Input: part model. Units: mm. Frame: model coordinates. A direction names the side the tool comes from. Give positions to 0.01 mm unless a question says otherwise; leave off trailing zeros. Loops run counter-clockwise (first coordinate to the right, second up) from the corner with the lowest first, then second, coordinate; pieces in that order, holes last. Notation, with made-up numbers: (19.5, 64) - (53.5, 64) arc R12 ccw to (53.5, 77) - close; hole circle Ø11 at (48, 52). An arc over 180 degrees is marked (long way). Answer as a JSON object with one key per item and string values. Group by question number.
(1) Access query for faces 4 (the cylindrical face through (-42.19, 15.07, -8.69)), 5 (the flat face through (-42, 15, 12)), 6 (the flat face through (-1, 2.5, 16)), 7 (the flat face through (27, 13.05, -27)). Directions: +Z, -Z, +X, -X, +Y, -Y. A direction counts if a zero-diameter tool reaches every point of the face in a straight line with its end or side. Return the directions, or none.
(2) Mould query, pull axis X, two halves, no side actions, for faces 1 (the flat face through (0, 6.5, 39)), 2 (the cylindrical face through (0.352, 14.93, -54.496)), 3 (the cylindrical face through (38.845, 7.918, -17.093)). Classes: +X half, -X half, draft (parallel to the pull), parting line (faces both ways), or undercut.
(3) Material intervals for L1, parallel to Z at x = 0, y = 1; L2, parallel to Z at x = -2, y = 18.25; L3, parallel to X at y = 9, z = 13, sorted ascending.
(4) Section query A-A (x = 0). Return loops of the section in (y, z).
(5) Section query B-B (z = -3.5). Return loops of the section in (x, y).
(6) Pin query (flat end, axial travel): P1, Ø2, axis at y = 11, z = -22, coming from the -X side; P2, Ø3, axis at x = 31, y = 15, coming from the +Z side; P3, Ø7.5, axis at x = 46, z = -6, coming from the -Y side. Return the tip coordinate at first contact, or that it passes through.
(7) Section query C-C (y = 5). Count the separate pieces of the cut face and the enclosed holes in it, plus the area to 3 significant figures.
```python
from build123d import *

# Parameters (mm, degrees)
BOSS_EXTRUDE1_DEPTH = 20
SKETCH5_W           = 4
SKETCH5_H           = 10
SKETCH16_W          = 2
SKETCH16_H          = 4.5
CUT_EXTRUDE9_DEPTH  = 10
SKETCH19_W          = 4
SKETCH19_H          = 10
CUT_EXTRUDE4_DEPTH  = 17.5
CUT_EXTRUDE5_DEPTH  = 2.5
SKETCH15_W          = 11.5
SKETCH15_H          = 4.5
CUT_EXTRUDE8_DEPTH  = 2.5
SKETCH17_W          = 14
SKETCH17_H          = 3
CUT_EXTRUDE10_DEPTH = 2.5
SKETCH21_W          = 4.5
SKETCH21_H          = 2
CUT_EXTRUDE11_DEPTH = 10
SKETCH22_R          = 2
CUT_EXTRUDE12_DEPTH = 2.5
FILLET1_R           = 10
FILLET2_R           = 4
SKETCH24_W          = 4.1
SKETCH24_H          = 4
CUT_EXTRUDE14_DEPTH = 77.5
SKETCH28_W          = 4.1
SKETCH28_H          = 4
CUT_EXTRUDE15_DEPTH = 77.5
SKETCH23_R          = 22.75
CUT_EXTRUDE13_DEPTH = 2.5


with BuildPart() as part:
    # Sketch1 → Boss-Extrude1 (new body)
    with BuildSketch(Plane(origin=(0, 0, 0), x_dir=(1, 0, 0), z_dir=(0, 1, 0))):
        Polygon((16.568542495, 40), (-16.568542495, 40), (-40, 16.568542495), (-40, -16.568542495), (-16.568542495, -40), (16.568542495, -40), (40, -16.568542495), (40, 16.568542495), align=None)
    extrude(amount=BOSS_EXTRUDE1_DEPTH)

    # Sweep9: sweep along a path in Sketch7
    with BuildLine(Plane(origin=(0, 15, 0), x_dir=(1, 0, 0), z_dir=(0, 1, 0))) as sweep9_path:
        ThreePointArc((40, -10.5), (50.5, 0), (40, 10.5))
    # Sketch5 → Sweep9 (sweep)
    with BuildSketch(Plane(origin=(40, 0, 0), x_dir=(0, 0, -1), z_dir=(1, 0, 0))):
        with Locations((-12.5, 15)):
            Rectangle(SKETCH5_W, SKETCH5_H)
        with Locations((12.5, 15)):
            Rectangle(SKETCH5_W, SKETCH5_H)
    sweep9 = sweep(path=sweep9_path.line)

    # Sketch16 → Cut-Extrude9 (cut)
    with BuildSketch(Plane(origin=(0, 20, 0), x_dir=(1, 0, 0), z_dir=(0, 1, 0))):
        with Locations((41, -12.25)):
            Rectangle(SKETCH16_W, SKETCH16_H)
    cut_extrude9 = extrude(amount=-CUT_EXTRUDE9_DEPTH, mode=Mode.SUBTRACT)

    # Mirror1: Sweep9, Cut-Extrude9 across plane
    add(sweep9.mirror(Plane(origin=(0, 0, 0), x_dir=(0, 0, 1), z_dir=(1, 0, 0))))
    add(cut_extrude9.mirror(Plane(origin=(0, 0, 0), x_dir=(0, 0, 1), z_dir=(1, 0, 0))), mode=Mode.SUBTRACT)

    # Sweep10: sweep along a path in Sketch20
    with BuildLine(Plane(origin=(0, 15, 0), x_dir=(1, 0, 0), z_dir=(0, 1, 0))) as sweep10_path:
        ThreePointArc((10.5, 40), (0, 50.5), (-10.5, 40))
    # Sketch19 → Sweep10 (sweep)
    with BuildSketch(Plane(origin=(0, 0, -40), x_dir=(-1, 0, 0), z_dir=(0, 0, -1))):
        with Locations((-12.5, 15)):
            Rectangle(SKETCH19_W, SKETCH19_H)
        with Locations((12.5, 15)):
            Rectangle(SKETCH19_W, SKETCH19_H)
    sweep(path=sweep10_path.line)

    # Sketch6 → Cut-Extrude4 (cut)
    with BuildSketch(Plane(origin=(0, 20, 0), x_dir=(1, 0, 0), z_dir=(0, 1, 0))):
        Polygon((-15.533008589, -37.5), (15.533008589, -37.5), (37.5, -15.533008589), (37.5, 15.533008589), (15.533008589, 37.5), (-15.533008589, 37.5), (-37.5, 15.533008589), (-37.5, -15.533008589), align=None)
    extrude(amount=-CUT_EXTRUDE4_DEPTH, mode=Mode.SUBTRACT)

    # Sketch3 → Cut-Extrude5 (cut)
    with BuildSketch(Plane.XY.offset(40)):
        with BuildLine():
            Line((-3.5, 6.5), (3.5, 6.5))
            ThreePointArc((3.5, 6.5), (5, 5), (3.5, 3.5))
            Line((3.5, 3.5), (-3.5, 3.5))
            ThreePointArc((-3.5, 3.5), (-5, 5), (-3.5, 6.5))
        make_face()
    extrude(amount=-CUT_EXTRUDE5_DEPTH, mode=Mode.SUBTRACT)

    # Sketch15 → Cut-Extrude8 (cut)
    with BuildSketch(Plane(origin=(28.284271247, 0, 28.284271247), x_dir=(0.707106781, 0, -0.707106781), z_dir=(0.707106781, 0, 0.707106781))):
        with Locations((0, 5)):
            Rectangle(SKETCH15_W, SKETCH15_H)
    extrude(amount=-CUT_EXTRUDE8_DEPTH, mode=Mode.SUBTRACT)

    # Sketch17 → Cut-Extrude10 (cut)
    with BuildSketch(Plane(origin=(-28.284271247, 0, 28.284271247), x_dir=(0.707106781, 0, 0.707106781), z_dir=(-0.707106781, 0, 0.707106781))):
        with Locations((0, 5)):
            Rectangle(SKETCH17_W, SKETCH17_H)
    extrude(amount=-CUT_EXTRUDE10_DEPTH, mode=Mode.SUBTRACT)

    # Sketch21 → Cut-Extrude11 (cut)
    with BuildSketch(Plane(origin=(0, 20, 0), x_dir=(1, 0, 0), z_dir=(0, 1, 0))):
        with Locations((12.25, 41)):
            Rectangle(SKETCH21_W, SKETCH21_H)
    extrude(amount=-CUT_EXTRUDE11_DEPTH, mode=Mode.SUBTRACT)

    # Sketch22 → Cut-Extrude12 (cut)
    with BuildSketch(Plane(origin=(28.284271247, 0, -28.284271247), x_dir=(-0.707106781, 0, -0.707106781), z_dir=(0.707106781, 0, -0.707106781))):
        with Locations((0, 10)):
            Circle(SKETCH22_R)
    extrude(amount=-CUT_EXTRUDE12_DEPTH, mode=Mode.SUBTRACT)

    # Fillet1
    fillet1_edges = [part.edges().sort_by_distance(p)[0] for p in [
        (-40, 10, -16.568542495),
        (-16.568542495, 10, -40),
        (16.568542495, 10, -40),
        (40, 10, -16.568542495),
        (-40, 10, 16.568542495),
        (40, 10, 16.568542495),
        (16.568542495, 10, 40),
        (-16.568542495, 10, 40),
    ]]
    fillet(fillet1_edges, radius=FILLET1_R)

    # Fillet2
    fillet2_edges = [part.edges().sort_by_distance(p)[0] for p in [
        (-10.5, 15, -40),
        (40, 15, -10.5),
        (-39.782992577, 15, -14.498376039),
        (-14.498376039, 15, -39.782992577),
        (39.782992577, 15, -14.498376039),
        (-40, 15, -10.5),
    ]]
    fillet(fillet2_edges, radius=FILLET2_R)

    # Sketch24 → Cut-Extrude14 (cut)
    with BuildSketch(Plane(origin=(-28.284271247, 0, 28.284271247), x_dir=(0.707106781, 0, 0.707106781), z_dir=(-0.707106781, 0, 0.707106781))):
        with Locations((0, 15.05)):
            Rectangle(SKETCH24_W, SKETCH24_H)
    cut_extrude14 = extrude(amount=-CUT_EXTRUDE14_DEPTH, mode=Mode.SUBTRACT)

    # Mirror2: Cut-Extrude14 across plane
    add(cut_extrude14.mirror(Plane(origin=(0, 0, 0), x_dir=(0.707106781, 0, 0.707106781), z_dir=(-0.707106781, 0, 0.707106781))), mode=Mode.SUBTRACT)

    # Sketch28 → Cut-Extrude15 (cut)
    with BuildSketch(Plane(origin=(28.284271247, 0, 28.284271247), x_dir=(0.707106781, 0, -0.707106781), z_dir=(0.707106781, 0, 0.707106781))):
        with Locations((0, 15.05)):
            Rectangle(SKETCH28_W, SKETCH28_H)
    cut_extrude15 = extrude(amount=-CUT_EXTRUDE15_DEPTH, mode=Mode.SUBTRACT)

    # Mirror3: Cut-Extrude15 across plane
    add(cut_extrude15.mirror(Plane(origin=(0, 0, 0), x_dir=(-0.707106781, 0, 0.707106781), z_dir=(0.707106781, 0, 0.707106781))), mode=Mode.SUBTRACT)

    # Sketch23 → Cut-Extrude13 (cut)
    with BuildSketch(Plane(origin=(0, 2.5, 0), x_dir=(1, 0, 0), z_dir=(0, 1, 0))):
        with Locations((0, 13)):
            Circle(SKETCH23_R)
    extrude(amount=-CUT_EXTRUDE13_DEPTH, mode=Mode.SUBTRACT)


solid = part.part
```
Recorded:
{
 "1": {"face 4": "+Y, -Y", "face 5": "+Z, +Y, -Y", "face 6": "+Y", "face 7": "none"},
 "2": {"face 1": "undercut", "face 2": "parting line", "face 3": "+X half"},
 "3": {"L1": "z = -40 to -35.75, 9.75 to 40", "L2": "z = -54.36 to -50.31, -40 to -37.5, 37.5 to 40", "L3": "x = -39.98 to -37.5, 37.5 to 39.98"},
 "4": {"outline": "(0, -40) - (20, -40) - (20, -37.5) - (2.5, -37.5) - (2.5, -35.75) - (0, -35.75) - close; (0, 9.75) - (2.5, 9.75) - (2.5, 37.5) - (3.5, 37.5) - (3.5, 40) - (0, 40) - close; (6.5, 37.5) - (20, 37.5) - (20, 40) - (6.5, 40) - close; (10, -54.5) - (20, -54.5) - (20, -50.5) - (10, -50.5) - close"},
 "5": {"outline": "(-54.07, 10) - (-49.9, 10) - (-49.9, 20) - (-54.07, 20) - close; (-40, 0) - (-20.67, 0) - (-20.67, 2.5) - (-37.5, 2.5) - (-37.5, 20) - (-40, 20) - close; (20.67, 0) - (40, 0) - (40, 20) - (37.5, 20) - (37.5, 2.5) - (20.67, 2.5) - close; (49.9, 10) - (54.07, 10) - (54.07, 20) - (49.9, 20) - close"},
 "6": {"P1": "stops at x = -35.57", "P2": "stops at z = 26.83", "P3": "stops at y = 10"},
 "7": {"separate pieces": "3", "enclosed holes": "0", "area": "536 mm^2"}
}
